Read the model definition and answer for the solid it produces. Units are mm, in the model's axes. A direction names the side the tool comes from. Give positions to 0.01 mm unless a question says otherwise; leave off trailing zeros. Loops run counter-clockwise (first coordinate to the right, second up) from the corner with the lowest first, then second, coordinate; pieces in that order, holes last. Notation, with made-up numbers: M -10.5,39.25 L -0.5,39.25 A19 cw -0.5,56.25 Z; hole C 34.25,86 d7. An arc over 180 degrees is marked long. Return JSON: item names as keys, results as strings. Group by question number.
```python
from build123d import *

# Parameters (mm, degrees)
BOSS_EXTRUDE3_DEPTH = 0.75
SKETCH6_R           = 0.75
BOSS_EXTRUDE4_DEPTH = 30


with BuildPart() as part:
    # Sketch2 → Boss-Extrude3 (new, symmetric)
    with BuildSketch(Plane(origin=(0, 0, 0), x_dir=(1, 0, 0), z_dir=(0, 1, 0))):
        with BuildLine():
            ThreePointArc((26.95, 0), (19.056527753, 19.056527753), (0, 26.95))
            Line((0, 26.95), (0, -26.95))
            ThreePointArc((0, -26.95), (19.056527753, -19.056527753), (26.95, 0))
        make_face()
        with BuildLine():
            Line((0, -26.95), (0, 26.95))
            ThreePointArc((0, 26.95), (-26.95, 0), (0, -26.95))
        make_face()
    extrude(amount=BOSS_EXTRUDE3_DEPTH, both=True)

    # Sketch6 → Boss-Extrude4 (add, symmetric)
    with BuildSketch(Plane(origin=(0, 0, 0), x_dir=(0, 0, -1), z_dir=(1, 0, 0))):
        with Locations(Location((0, 0, 0), (0, 0, 90))):
            Circle(SKETCH6_R)
    extrude(amount=BOSS_EXTRUDE4_DEPTH, both=True)


solid = part.part
```
1. Find section C-C (z = -2). Write down the section's boundary in (x, y).
2. Find section B-B (x = -21.5). Write down the section's boundary in (y, z), and give its area (3 significant figures).
3. Straight lines are drawn through the part: line 1 along X through (y, z) = (-0.05, 1); line 2 along Z through (x, y) = (14.5, -0.2); line 3 along X through (y, z) = (0.15, 19). For each, find the intervals that lie inside material, in ascending order.
4. For faces 1 (the cylindrical face through (28.491, 0.715, 0.225)), 2 (the cylindrical face through (-28.448, 0.715, 0.225)), 3 (the flat face through (30, 0, 0)), determine the directions among +Z, -Z, +X, -X, +Y, -Y from which every point of the face is accessible in a straight line to the end or side of a thin tool.
Result:
{
 "1": {"outline": "M -26.88,-0.75 L 26.88,-0.75 L 26.88,0.75 L -26.88,0.75 Z"},
 "2": {"outline": "M -0.75,-16.25 L 0.75,-16.25 L 0.75,16.25 L -0.75,16.25 Z", "area": "48.7 mm2"},
 "3": {"line 1": "x = -26.93 to 26.93", "line 2": "z = -22.72 to 22.72", "line 3": "x = -19.11 to 19.11"},
 "4": {"face 1": "+X", "face 2": "-X", "face 3": "+Z, -Z, +X, +Y, -Y"}
}
